Can you work these out from the model? Positions are in its coordinate system, mm. A direction names the side the tool comes from. Round coordinates to 2 decimals unless told otherwise and drop trailing zeros. Write each loop counter-clockwise with the first axis right and the second up, starting at its lowest first coordinate (ties: lowest second). Pieces come first, ordered by that corner, then holes. Notation, with made-up numbers: M -19.5,21 L -14.5,21 A15 ccw -14.5,40 Z; hole C -27.75,44.25 d1. An arc over 180 degrees is marked long. Use one line per item in the form item = value. Start each with the question number.
```python
from build123d import *

# Parameters (mm, degrees)
ESQUISSE3_W             = 80
ESQUISSE3_H             = 10
EXTRU_MINCE4_DEPTH      = 100
ESQUISSE4_W             = 2
ESQUISSE4_H             = 100
ENL_V_MAT_EXTRU_1_DEPTH = 0.6
ENL_V_MAT_EXTRU_2_DEPTH = 11
ESQUISSE6_W             = 80
ESQUISSE6_H             = 100
BOSS_EXTRU_1_DEPTH      = 3


with BuildPart() as part:
    # Esquisse3 → Extru.-Mince4 (new body)
    with BuildSketch(Plane.XY):
        with Locations((0, -5)):
            Rectangle(ESQUISSE3_W, ESQUISSE3_H)
    extrude(amount=EXTRU_MINCE4_DEPTH)

    # Esquisse4 → Enlèv. mat.-Extru.1 (cut)
    with BuildSketch(Plane(origin=(0, 0, 0), x_dir=(1, 0, 0), z_dir=(0, 1, 0))):
        with Locations((-34, -50)):
            Rectangle(ESQUISSE4_W, ESQUISSE4_H)
        with Locations((34, -50)):
            Rectangle(ESQUISSE4_W, ESQUISSE4_H)
    extrude(amount=-ENL_V_MAT_EXTRU_1_DEPTH, mode=Mode.SUBTRACT)

    # Esquisse5 → Enlèv. mat.-Extru.2 (cut)
    with BuildSketch(Plane(origin=(0, 0, 0), x_dir=(1, 0, 0), z_dir=(0, 1, 0))):
        Polygon((0, 0), (-8, 0), (-8, -100), (8, -100), (8, 0), align=None)
    extrude(amount=-ENL_V_MAT_EXTRU_2_DEPTH, mode=Mode.SUBTRACT)

    # Esquisse6 → Boss.-Extru.1 (add)
    with BuildSketch(Plane.XZ.offset(10)):
        with Locations((0, 50)):
            Rectangle(ESQUISSE6_W, ESQUISSE6_H)
    extrude(amount=BOSS_EXTRU_1_DEPTH)


solid = part.part
```
1. Will these pins go through, and if not, where does the flat tip stop? pin 1 (0.6 mm diameter, centred on x = 34, z = 68.5, fed in from +Y); pin 2 (4 mm diameter, centred on x = -2.5, z = 33, fed in from +Y).
2. Please list where these lines run through material, in increasing order: line 1 along X through (y, z) = (-1.75, 43); line 2 along Y through (x, z) = (-7, 70).
3. If we section it at C-C (x = 5): List the corners of the cut face in (y, z) for me.
4. Which directions (+Z, -Z, +X, -X, +Y, -Y) give clear straight access to the entire face, cutting with the end or side of a thin tool? Please do faces 1 (the face through (-34, -0.6, 49)), 2 (the face through (-21, 0, 49)).
5. If we section it at B-B (z = 32.5): List the corners of the cut face in (x, y) for me, and give its area (3 significant figures).
6. If we mould it in two halves opening along X, with no side actions, what happens to faces 3 (the face through (-8, -5, 49)), 4 (the face through (-40, -6, 49)), 5 (the face through (-1, -11, 0))? For each: pulls with the +X half, pulls with the -X half, needs draft (parallel to the pull), parting line crosses it, or undercut.
7. If we section it at A-A (y = -3.75): List the corners of the cut face in (x, z) for me, and give its area (3 significant figures).
Model answer:
q1.pin_1 = -0.6
q1.pin_2 = -10
q2.line_1 = -40 to -8, 8 to 40
q2.line_2 = -13 to -10
q3.outline = M -13,0 L -10,0 L -10,100 L -13,100 Z
q4.face_1 = +Z, -Z, +Y
q4.face_2 = +Z, -Z, +X, -X, +Y
q5.outline = M -40,-13 L 40,-13 L 40,0 L 35,0 L 35,-0.6 L 33,-0.6 L 33,0 L 8,0 L 8,-10 L -8,-10 L -8,0 L -33,0 L -33,-0.6 L -35,-0.6 L -35,0 L -40,0 Z
q5.area = 878 mm2
q6.face_3 = undercut
q6.face_4 = pulls with the -X half
q6.face_5 = needs draft
q7.outline = M -40,0 L -8,0 L -8,100 L -40,100 Z; M 8,0 L 40,0 L 40,100 L 8,100 Z
q7.area = 6,400 mm2
